Input: part model. Units: mm. Frame: model coordinates. A direction names the side the tool comes from. Give positions to 0.01 mm unless a question says otherwise; leave off trailing zeros. Loops run counter-clockwise (first coordinate to the right, second up) from the corner with the lowest first, then second, coordinate; pieces in that order, holes last. Notation, with made-up numbers: (57.25, -11) -> (113.25, -11) arc R15 ccw to (113.25, -6) -> close; hole circle Ø2 at (16.25, -35.75). An arc over 180 degrees is marked (long way). Answer as a JSON object with one key per item and string values.
```python
from build123d import *

# Parameters (mm, degrees)
SKETCH1_R             = 0.5
BOSS_EXTRUDE1_DEPTH   = 8
M3_CLEARANCE_HOLE1_D  = 3.4
M3X0_5_TAPPED_HOLE1_D = 2.5
SKETCH6_W             = 67.2
SKETCH6_H             = 8
CUT_EXTRUDE1_DEPTH    = 0.25


with BuildPart() as part:
    # Sketch1 → Boss-Extrude1 (new body)
    with BuildSketch(Plane.XY):
        with BuildLine():
            Line((-33.6, 0), (33.6, 0))
            Line((33.6, 0), (33.6, 2.345845935))
            ThreePointArc((33.6, 2.345845935), (33.913217108, 3.420445152), (34.754763477, 4.158461509))
            Line((34.754763477, 4.158461509), (48.856545654, 10.734230532))
            ThreePointArc((48.856545654, 10.734230532), (50.188323304, 13.73885844), (47.392535439, 15.466571027))
            Line((47.392535439, 15.466571027), (34.889574734, 13.401147676))
            ThreePointArc((34.889574734, 13.401147676), (32.45300125, 13.100455106), (30, 13))
            Line((30, 13), (-30, 13))
            ThreePointArc((-30, 13), (-32.45300125, 13.100455106), (-34.889574734, 13.401147676))
            Line((-34.889574734, 13.401147676), (-47.392535439, 15.466571027))
            ThreePointArc((-47.392535439, 15.466571027), (-50.188323304, 13.73885844), (-48.856545654, 10.734230532))
            Line((-48.856545654, 10.734230532), (-34.754763477, 4.158461509))
            ThreePointArc((-34.754763477, 4.158461509), (-33.913217108, 3.420445152), (-33.6, 2.345845935))
            Line((-33.6, 2.345845935), (-33.6, 0))
        make_face()
        with Locations((-47.8, 13)):
            Circle(SKETCH1_R, mode=Mode.SUBTRACT)
        with Locations((47.8, 13)):
            Circle(SKETCH1_R, mode=Mode.SUBTRACT)
        with Locations((-44.041229517, 11.631919427)):
            Circle(SKETCH1_R, mode=Mode.SUBTRACT)
        with Locations((44.041229517, 11.631919427)):
            Circle(SKETCH1_R, mode=Mode.SUBTRACT)
        with BuildLine():
            Line((33, 8.75), (33, 9.25))
            ThreePointArc((33, 9.25), (32.707106781, 9.957106781), (32, 10.25))
            Line((32, 10.25), (-32, 10.25))
            ThreePointArc((-32, 10.25), (-32.707106781, 9.957106781), (-33, 9.25))
            Line((-33, 9.25), (-33, 8.75))
            ThreePointArc((-33, 8.75), (-32.707106781, 8.042893219), (-32, 7.75))
            Line((-32, 7.75), (32, 7.75))
            ThreePointArc((32, 7.75), (32.707106781, 8.042893219), (33, 8.75))
        make_face(mode=Mode.SUBTRACT)
    extrude(amount=BOSS_EXTRUDE1_DEPTH)

    # M3 Clearance Hole1 (through all)
    with Locations(Plane.XY.offset(8)):
        with Locations((-17.5, 3.5), (17.5, 3.5)):
            Hole(M3_CLEARANCE_HOLE1_D / 2)

    # M3x0.5 Tapped Hole1 (through all)
    with Locations(Plane.XY.offset(8)):
        with Locations((-47.8, 13), (47.8, 13), (-44.041229517, 11.631919427), (44.041229517, 11.631919427)):
            Hole(M3X0_5_TAPPED_HOLE1_D / 2)

    # Sketch6 → Cut-Extrude1 (cut)
    with BuildSketch(Plane.XZ):
        with Locations((0, 4)):
            Rectangle(SKETCH6_W, SKETCH6_H)
    extrude(amount=-CUT_EXTRUDE1_DEPTH, mode=Mode.SUBTRACT)


solid = part.part
```
Q1. Draft query along X for faces 4 (the cylindrical face through (-42.792, 11.687, 3.944)), 5 (the flat face through (-1, 6, 0)), 6 (the cylindrical face through (-19.07, 2.85, 3.94)), 7 (the flat face through (-41.9, 7.49, 3.94)). Return one class per face: +X half, -X half, draft (parallel to the pull), parting line (faces both ways), or undercut.
Evaluation:
{"face 4": "undercut", "face 5": "draft", "face 6": "undercut", "face 7": "-X half"}
Q2. Ray query, line 1 along Y through (x, z) = (17.5, 2); line 2 along Y through (x, z) = (11, 6.5); line 3 along X through (y, z) = (11.25, 6.5). Return the intervals inside material, ascending.
Evaluation:
{"line 1": "y = 0.25 to 1.8, 5.2 to 7.75, 10.25 to 13", "line 2": "y = 0.25 to 7.75, 10.25 to 13", "line 3": "x = -49.59 to -45.23, -42.85 to 42.85, 45.23 to 49.59"}
Q3. Pin query (flat end, axial travel): pin 1 (1.5 mm diameter, centred on y = 11.5, z = 5.5, fed in from +X); pin 2 (4 mm diameter, centred on x = -47.8, y = 13, fed in from -Z); pin 3 (0.6 mm diameter, centred on y = 1, z = 4.5, fed in from +X); pin 4 (2.5 mm diameter, centred on y = 1, z = 2.5, fed in from -X). Return the tip coordinate at first contact, or that it passes through.
Evaluation:
{"pin 1": "stops at x = 50.18", "pin 2": "stops at z = 0", "pin 3": "stops at x = 33.6", "pin 4": "stops at x = -33.6"}
Q4. Section B-B, the plane z = 1. Return the cut outline in (x, y), then the cut area to 3 significant figures.
Evaluation:
{"outline": "(-48.86, 10.73) -> (-34.75, 4.16) arc R2 cw to (-33.6, 2.35) -> (-33.6, 0.25) -> (33.6, 0.25) -> (33.6, 2.35) arc R2 cw to (34.75, 4.16) -> (48.86, 10.73) arc R2.5 ccw to (47.39, 15.47) -> (34.89, 13.4) arc R30 cw to (30, 13) -> (-30, 13) arc R30 cw to (-34.89, 13.4) -> (-47.39, 15.47) arc R2.5 ccw to start; hole circle Ø2.5 at (-47.8, 13); hole circle Ø2.5 at (-44.04, 11.63); hole (-33, 8.75) arc R1 ccw to (-32, 7.75) -> (32, 7.75) arc R1 ccw to (33, 8.75) -> (33, 9.25) arc R1 ccw to (32, 10.25) -> (-32, 10.25) arc R1 ccw to (-33, 9.25) -> close; hole circle Ø3.4 at (-17.5, 3.5); hole circle Ø3.4 at (17.5, 3.5); hole circle Ø2.5 at (44.04, 11.63); hole circle Ø2.5 at (47.8, 13)", "area": "887 mm2"}
Q5. Section A-A, the plane x = -17.5. Return the cut outline in (y, z).
Evaluation:
{"outline": "(0.25, 0) -> (1.8, 0) -> (1.8, 8) -> (0.25, 8) -> close; (5.2, 0) -> (7.75, 0) -> (7.75, 8) -> (5.2, 8) -> close; (10.25, 0) -> (13, 0) -> (13, 8) -> (10.25, 8) -> close"}
Q6. Access query for faces 1 (the flat face through (-33.6, 1, 4)), 2 (the flat face through (0, 10.25, 4)), 3 (the flat face through (0, 13, 4)). Directions: +Z, -Z, +X, -X, +Y, -Y. A direction counts if a zero-diameter tool reaches every point of the face in a straight line with its end or side. Return the directions, or none.
Evaluation:
{"face 1": "+Z, -Z, -X, -Y", "face 2": "+Z, -Z", "face 3": "+Z, -Z, +Y"}
